from build123d import *

# Parameters (mm, degrees)
SKETCH_1_R               = 6
EXTRUDE_2_DEPTH          = 150
CUT_EXTRUDE_2_DEPTH      = 151.239808307
CUT_EXTRUDE_2_DEPTH_BACK = 18
SKETCH_3_R               = 3
CUT_EXTRUDE_4_REACH      = 152.24
CUT_EXTRUDE_4_END_RADIUS = 6
SKETCH_4_R               = 1.25
SKETCH_5_R               = 6
SKETCH_5_R_2             = 5
CUT_EXTRUDE_5_DEPTH      = 15


with BuildPart() as part:
    # ｽｹｯﾁ1 → ﾎﾞｽ - 押し出し2 (new body)
    with BuildSketch(Plane(origin=(0, 0, 0), x_dir=(1, 0, 0), z_dir=(0, 1, 0))):
        with Locations(Location((0, 0, 0), (0, 0, 270))):
            Circle(SKETCH_1_R)
    extrude(amount=EXTRUDE_2_DEPTH)

    # ｽｹｯﾁ3 → ｶｯﾄ - 押し出し2 (cut, two sides: drawn at the far end of the back side and taken through both)
    with BuildSketch(Plane(origin=(0, 150, 0), x_dir=(1, 0, 0), z_dir=(0, 1, 0)).offset(-CUT_EXTRUDE_2_DEPTH_BACK)):
        with Locations(Location((0, 0, 0), (0, 0, 90))):
            Circle(SKETCH_3_R)
    extrude(amount=CUT_EXTRUDE_2_DEPTH + CUT_EXTRUDE_2_DEPTH_BACK, mode=Mode.SUBTRACT)

    # ｶｯﾄ - 押し出し4: up to this cylinder (the profile starts inside it)
    cut_extrude_4_end = Plane(origin=(0, 142, 0), z_dir=(0, -1, 0)) * Cylinder(CUT_EXTRUDE_4_END_RADIUS, 317.48, mode=Mode.PRIVATE)
    # ｽｹｯﾁ4 → ｶｯﾄ - 押し出し4 (cut, up to the surface)
    with BuildSketch(Plane.XY, mode=Mode.PRIVATE) as cut_extrude_4_sk1:
        with Locations((0, 142)):
            Circle(SKETCH_4_R)
    cut_extrude_4_tool1 = extrude(cut_extrude_4_sk1.sketch, amount=-CUT_EXTRUDE_4_REACH, mode=Mode.PRIVATE) & cut_extrude_4_end
    add(cut_extrude_4_tool1.solids().sort_by_distance((0, 142, 0))[0], mode=Mode.SUBTRACT)

    # ｽｹｯﾁ5 → ｶｯﾄ - 押し出し5 (cut)
    with BuildSketch(Plane.XZ):
        with Locations(Location((0, 0, 0), (0, 0, 270))):
            Circle(SKETCH_5_R)
        with Locations(Location((0, 0, 0), (0, 0, 270))):
            Circle(SKETCH_5_R_2, mode=Mode.SUBTRACT)
    extrude(amount=-CUT_EXTRUDE_5_DEPTH, mode=Mode.SUBTRACT)


solid = part.part
Input: part model. Units: mm. Frame: model coordinates. A direction names the side the tool comes from. Coordinates: 2 decimals unless noted, no trailing zeros. Loops run counter-clockwise (first coordinate to the right, second up) from the corner with the lowest first, then second, coordinate; pieces in that order, holes last. Notation, with made-up numbers: (21, 34.5) - (53, 34.5) arc R14 ccw to (53, 43.5) - close; hole circle Ø8 at (17.5, -25). An arc over 180 degrees is marked (long way). Answer in a Markdown table with one row per item. Add a question column.
Item 1: Mould query, pull axis Z, two halves, no side actions, for faces 1 (the cylindrical face through (-4.88, 7.4, 1.08)), 2 (the flat face through (0, 132, 0)), 3 (the cylindrical face through (-0.9, 140.87, -2.86)), 4 (the cylindrical face through (-1.25, 142.05, -4.34)). Classes: released by +Z, released by -Z, zero draft, split by the parting line, or undercut.
Item 2: Line query: line 1 along X through (y, z) = (138, 0); line 2 along Y through (x, z) = (4.75, 1.75); line 3 along Y through (x, z) = (-0.5, -4.5). Output: solid intervals per line, ascending. Write a range as [from, to].
Item 3: Access query for faces 5 (the flat face through (4, 15, 4)), 6 (the flat face through (0, 0, 0)). Directions: +Z, -Z, +X, -X, +Y, -Y. A direction counts if a zero-diameter tool reaches every point of the face in a straight line with its end or side. Return the directions, or none.
Item 4: Section query A-A on x = 0. Return the cut outline in (y, z).
Item 5: Section query C-C on y = 65. Return the cut outline in (x, z).
Item 6: Contact query for flat-ended pins moving along their axis: P1, Ø2, axis at y = 114, z = 4, coming from the -X side; P2, Ø1.5, axis at x = -0.5, z = 0, coming from the +Y side; P3, Ø6, axis at y = 72, z = 3.5, coming from the -X side. Output: stop coordinate, or through.
Item 7: Section query D-D on y = 11. Return the cut outline in (x, z), then the cut area to 3 significant figures.
Item 8: Section query B-B on z = 0. Return the cut outline in (x, y).
Recorded:
| question | item | result |
|---|---|---|
| 1 | face 1 | split by the parting line |
| 1 | face 2 | undercut |
| 1 | face 3 | undercut |
| 1 | face 4 | zero draft |
| 2 | line 1 | [-6, -3], [3, 6] |
| 2 | line 2 | [15, 150] |
| 2 | line 3 | [0, 140.85], [143.15, 150] |
| 3 | face 5 | -Y |
| 3 | face 6 | +Z, -Z, +X, -X, -Y |
| 4 | outline | (0, -5) - (15, -5) - (15, -6) - (140.75, -6) - (140.75, -3) - (132, -3) - (132, 3) - (150, 3) - (150, 6) - (15, 6) - (15, 5) - (0, 5) - close; (143.25, -6) - (150, -6) - (150, -3) - (143.25, -3) - close |
| 5 | outline | circle Ø12 at (0, 0) |
| 6 | P1 | x = -5.2 |
| 6 | P2 | y = 132 |
| 6 | P3 | x = -5.98 |
| 7 | outline | circle Ø10 at (0, 0) |
| 7 | area | 78.5 mm^2 |
| 8 | outline | (-6, 15) - (-5, 15) - (-5, 0) - (5, 0) - (5, 15) - (6, 15) - (6, 150) - (3, 150) - (3, 132) - (-3, 132) - (-3, 150) - (-6, 150) - close |
